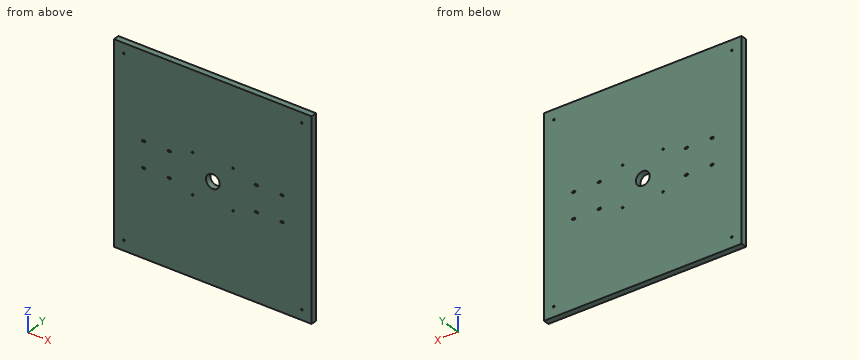
```python
from build123d import *

# Parameters (mm, degrees)
CROQUIS1_W              = 500
CROQUIS1_H              = 500
SALIENTE_EXTRUIR1_DEPTH = 15
CROQUIS2_R              = 2.15
CORTAR_EXTRUIR1_DEPTH   = 15
CROQUIS3_R              = 2.15
CORTAR_EXTRUIR3_DEPTH   = 15
CROQUIS4_R              = 17.5
CORTAR_EXTRUIR4_DEPTH   = 40


with BuildPart() as part:
    # Croquis1 → Saliente-Extruir1 (new body)
    with BuildSketch(Plane(origin=(0, 0, 0), x_dir=(1, 0, 0), z_dir=(0, 1, 0))):
        Rectangle(CROQUIS1_W, CROQUIS1_H)
    extrude(amount=SALIENTE_EXTRUIR1_DEPTH)

    # Croquis2 → Cortar-Extruir1 (cut)
    with BuildSketch(Plane(origin=(0, 15, 0), x_dir=(1, 0, 0), z_dir=(0, 1, 0))):
        with Locations(Location((-225, 225, 0), (0, 0, 270))):
            Circle(CROQUIS2_R)
        with Locations(Location((225, 225, 0), (0, 0, 90))):
            Circle(CROQUIS2_R)
        with Locations(Location((225, -225, 0), (0, 0, 270))):
            Circle(CROQUIS2_R)
        with Locations(Location((-225, -225, 0), (0, 0, 90))):
            Circle(CROQUIS2_R)
    extrude(amount=-CORTAR_EXTRUIR1_DEPTH, mode=Mode.SUBTRACT)

    # Croquis3 → Cortar-Extruir3 (cut)
    with BuildSketch(Plane(origin=(0, 15, 0), x_dir=(1, 0, 0), z_dir=(0, 1, 0))):
        with Locations(Location((-51.265, 51.265, 0), (0, 0, 270))):
            Circle(CROQUIS3_R)
        with Locations(Location((-51.265, -51.265, 0), (0, 0, 270))):
            Circle(CROQUIS3_R)
        with Locations(Location((51.265, -51.265, 0), (0, 0, 270))):
            Circle(CROQUIS3_R)
        with Locations(Location((51.265, 51.265, 0), (0, 0, 270))):
            Circle(CROQUIS3_R)
        with BuildLine():
            Line((-177.115, 34.55), (-172.815, 34.55))
            ThreePointArc((-172.815, 34.55), (-170.665, 32.4), (-172.815, 30.25))
            Line((-172.815, 30.25), (-177.115, 30.25))
            ThreePointArc((-177.115, 30.25), (-179.265, 32.4), (-177.115, 34.55))
        make_face()
        with BuildLine():
            Line((-177.115, -30.25), (-172.815, -30.25))
            ThreePointArc((-172.815, -30.25), (-170.665, -32.4), (-172.815, -34.55))
            Line((-172.815, -34.55), (-177.115, -34.55))
            ThreePointArc((-177.115, -34.55), (-179.265, -32.4), (-177.115, -30.25))
        make_face()
        with BuildLine():
            Line((-112.315, -30.25), (-108.015, -30.25))
            ThreePointArc((-108.015, -30.25), (-105.865, -32.4), (-108.015, -34.55))
            Line((-108.015, -34.55), (-112.315, -34.55))
            ThreePointArc((-112.315, -34.55), (-114.465, -32.4), (-112.315, -30.25))
        make_face()
        with BuildLine():
            Line((-112.315, 34.55), (-108.015, 34.55))
            ThreePointArc((-108.015, 34.55), (-105.865, 32.4), (-108.015, 30.25))
            Line((-108.015, 30.25), (-112.315, 30.25))
            ThreePointArc((-112.315, 30.25), (-114.465, 32.4), (-112.315, 34.55))
        make_face()
        with BuildLine():
            Line((177.115, -30.25), (172.815, -30.25))
            ThreePointArc((172.815, -30.25), (170.665, -32.4), (172.815, -34.55))
            Line((172.815, -34.55), (177.115, -34.55))
            ThreePointArc((177.115, -34.55), (179.265, -32.4), (177.115, -30.25))
        make_face()
        with BuildLine():
            Line((177.115, 34.55), (172.815, 34.55))
            ThreePointArc((172.815, 34.55), (170.665, 32.4), (172.815, 30.25))
            Line((172.815, 30.25), (177.115, 30.25))
            ThreePointArc((177.115, 30.25), (179.265, 32.4), (177.115, 34.55))
        make_face()
        with BuildLine():
            Line((112.315, -30.25), (108.015, -30.25))
            ThreePointArc((108.015, -30.25), (105.865, -32.4), (108.015, -34.55))
            Line((108.015, -34.55), (112.315, -34.55))
            ThreePointArc((112.315, -34.55), (114.465, -32.4), (112.315, -30.25))
        make_face()
        with BuildLine():
            Line((112.315, 34.55), (108.015, 34.55))
            ThreePointArc((108.015, 34.55), (105.865, 32.4), (108.015, 30.25))
            Line((108.015, 30.25), (112.315, 30.25))
            ThreePointArc((112.315, 30.25), (114.465, 32.4), (112.315, 34.55))
        make_face()
    extrude(amount=-CORTAR_EXTRUIR3_DEPTH, mode=Mode.SUBTRACT)

    # Croquis4 → Cortar-Extruir4 (cut)
    with BuildSketch(Plane(origin=(0, 15, 0), x_dir=(1, 0, 0), z_dir=(0, 1, 0))):
        with Locations(Location((0, 0, 0), (0, 0, 270))):
            Circle(CROQUIS4_R)
    extrude(amount=-CORTAR_EXTRUIR4_DEPTH, mode=Mode.SUBTRACT)


solid = part.part
```
Model file for the job. Use its own axes, mm. Give positions to 0.01 mm unless a question says otherwise; leave off trailing zeros. Order: outer loops, then holes, each group sorted by start corner. A loop starts at its lowest first (then second) coordinate and runs counter-clockwise, first axis right, second up.
1) Saw through at A-A, the plane z = 0. Write the cut outline in (x, y).
2) Wall check: probe 1 along Z at (x, y) = (-107.5, 3.5); probe 2 along Z at (x, y) = (-225, 10.5); probe 3 along Z at (x, y) = (-6.5, 4). Give the ranges that are in metal, low to high.
3) Pin check, flat tips, straight feed: pin 1 (2.5 mm diameter, centred on x = -225, z = 225, fed in from +Y); pin 2 (5 mm diameter, centred on x = -51.265, z = -51.265, fed in from +Y). Stop position of each tip, or through.
Computed:
1. outline: (-250, 0) - (-17.5, 0) - (-17.5, 15) - (-250, 15) - close; (17.5, 0) - (250, 0) - (250, 15) - (17.5, 15) - close
2. probe 1: z = -250 to -34.49, -30.31 to 30.31, 34.49 to 250
2. probe 2: z = -250 to -227.15, -222.85 to 222.85, 227.15 to 250
2. probe 3: z = -250 to -16.25, 16.25 to 250
3. pin 1: passes through
3. pin 2: stops at y = 15
